Geometry check sheet. Reference: drawing and pictorial views, mm from the part's lowest x, y, z. Coordinates: 2 decimals unless noted, no trailing zeros. Loops run counter-clockwise (first coordinate to the right, second up) from the corner with the lowest first, then second, coordinate; pieces in that order, holes last. Notation, with made-up numbers: (11, -39) -> (34, -39) arc R21 ccw to (34, -23) -> close; hole circle Ø8 at (7, 2). An arc over 180 degrees is marked (long way). Answer as a JSON object with one key per item and string values. Group by question number.
Q1. Gauge pin test, flat ends, axial feed: pin 1 Ø3 at (y, z) = (5.5, 131) entering from -X; pin 2 Ø0.9 at (x, y) = (15.5, 5.5) entering from -Z; pin 3 Ø1.5 at (x, y) = (15, 4.5) entering from +Z; pin 4 Ø5.5 at (x, z) = (55, 10) entering from -Y. Record the tip position at first contact, or that the pin passes through.
Q2. Cross-section at C-C on y = 1.75. Record the boundary of the cut face in (x, z), and give its area (3 significant figures).
Q3. Cross-section at A-A on z = 270. Record the boundary of the cut face in (x, y).
Q4. Cross-section at D-D on x = 30.5. Record the boundary of the cut face in (y, z).
Q5. Cross-section at B-B on z = 200. Record the boundary of the cut face in (x, y).
Q6. Scan lines: L1, parallel to X at y = 3, z = 80; L2, parallel to X at y = 3, z = 140; L3, parallel to X at y = 4, z = 10. Record each from-to range of solid material in increasing order.
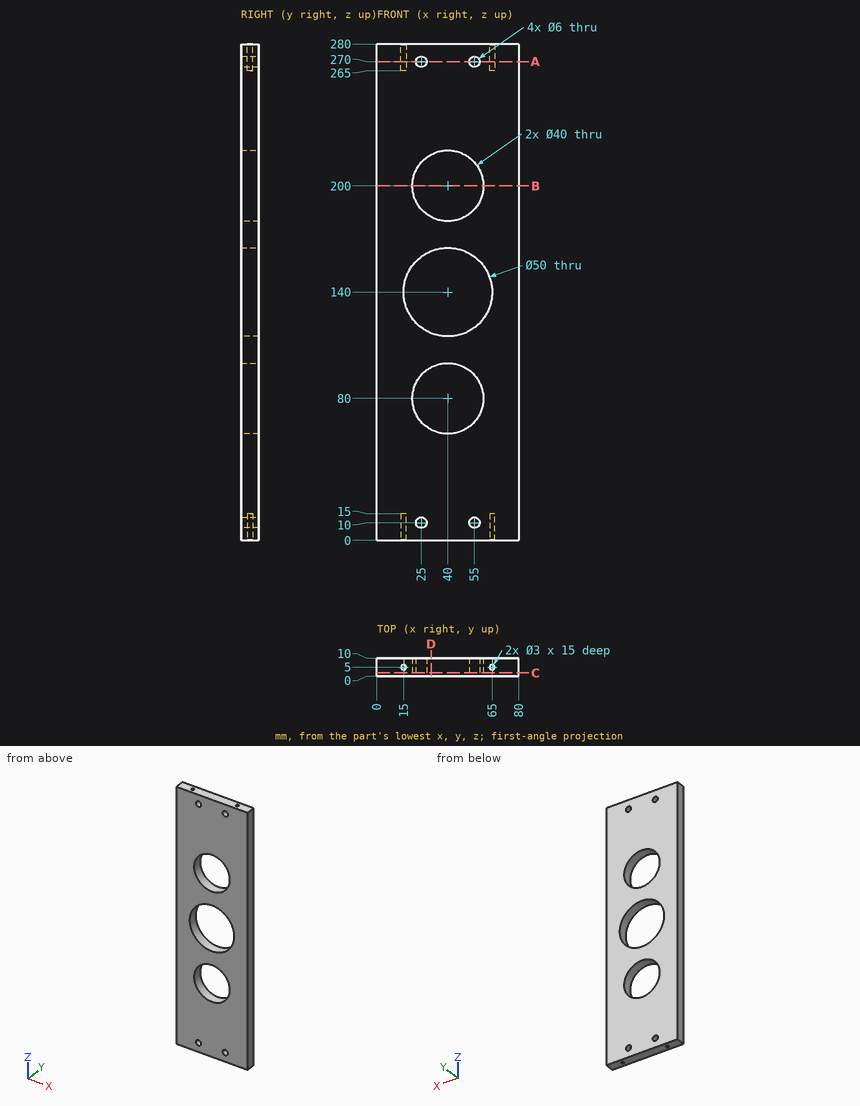
Computed values:
{
 "1": {"pin 1": "stops at x = 0", "pin 2": "stops at z = 15", "pin 3": "stops at z = 265", "pin 4": "passes through"},
 "2": {"outline": "(0, 0) -> (80, 0) -> (80, 280) -> (0, 280) -> close; hole circle Ø50 at (40, 140); hole circle Ø40 at (40, 80); hole circle Ø40 at (40, 200); hole circle Ø6 at (25, 10); hole circle Ø6 at (25, 270); hole circle Ø6 at (55, 10); hole circle Ø6 at (55, 270)", "area": "17,800 mm²"},
 "3": {"outline": "(0, 0) -> (22, 0) -> (22, 10) -> (0, 10) -> close; (28, 0) -> (52, 0) -> (52, 10) -> (28, 10) -> close; (58, 0) -> (80, 0) -> (80, 10) -> (58, 10) -> close; hole circle Ø3 at (15, 5); hole circle Ø3 at (65, 5)"},
 "4": {"outline": "(0, 0) -> (10, 0) -> (10, 62.4) -> (0, 62.4) -> close; (0, 97.6) -> (10, 97.6) -> (10, 116.88) -> (0, 116.88) -> close; (0, 163.12) -> (10, 163.12) -> (10, 182.4) -> (0, 182.4) -> close; (0, 217.6) -> (10, 217.6) -> (10, 280) -> (0, 280) -> close"},
 "5": {"outline": "(0, 0) -> (20, 0) -> (20, 10) -> (0, 10) -> close; (60, 0) -> (80, 0) -> (80, 10) -> (60, 10) -> close"},
 "6": {"L1": "x = 0 to 20, 60 to 80", "L2": "x = 0 to 15, 65 to 80", "L3": "x = 0 to 13.88, 16.12 to 22, 28 to 52, 58 to 63.88, 66.12 to 80"}
}
